from build123d import *

# Parameters (mm, degrees)
CHAMFER1_SIZE = 0.5


with BuildPart() as part:
    # Sketch1 → Revolve1 (revolve)
    with BuildSketch(Plane.XY, mode=Mode.PRIVATE) as revolve1_sk:
        with BuildLine():
            Line((5.5, 10.5), (2.236067977, 10.5))
            ThreePointArc((2.236067977, 10.5), (0, 9.5), (-2.236067977, 10.5))
            Line((-2.236067977, 10.5), (-5.5, 10.5))
            Line((-5.5, 10.5), (-5.5, 7.5))
            Line((-5.5, 7.5), (5.5, 7.5))
            Line((5.5, 7.5), (5.5, 10.5))
        make_face()
    revolve(revolve1_sk.sketch.rotate(Axis((-28.291139241, 0, 0), (1, 0, 0)), 90), axis=Axis((-28.291139241, 0, 0), (1, 0, 0)))

    # Chamfer1
    chamfer1_edges = [part.edges().sort_by_distance(p)[0] for p in [
        (-5.5, 0, -10.5),
        (5.5, 0, -10.5),
        (5.5, 0, -7.5),
        (-5.5, 0, -7.5),
    ]]
    chamfer(chamfer1_edges, length=CHAMFER1_SIZE)


solid = part.part
The listing builds one solid part. Answer for the finished solid, in the listing's coordinates (mm). Round coordinates to 2 decimals unless told otherwise and drop trailing zeros. Order: outer loops, then holes, each group sorted by start corner. A loop starts at its lowest first (then second) coordinate and runs counter-clockwise, first axis right, second up. Notation, with made-up numbers: M -10,45.25 L 24,45.25 A13 cw 24,62.25 Z; hole C -7.75,23.25 d7. An arc over 180 degrees is marked long. Answer in a Markdown table with one row per item. Add a question column.
1) The part is cut by section A-A on z = 0. Determine the outline of the cut face in (x, y).
2) Flat-ended cylindrical pins translate along their axes: pin 1 Ø10 at (y, z) = (-2.5, 5) entering from +X; pin 2 Ø2 at (x, z) = (-1.5, 5.5) entering from -Y; pin 3 Ø1 at (x, y) = (-3, 3.5) entering from +Z; pin 4 Ø1 at (x, z) = (-1.5, 1.5) entering from -Y. Find the tip coordinate at first contact, or state that the pin passes through.
3) The part is cut by section C-C on x = 1.25. Determine the outline of the cut face in (y, z), plus the area to 3 significant figures.
4) The part is cut by section B-B on x = -3.5. Determine the outline of the cut face in (y, z), plus the area to 3 significant figures.
5) Determine the mould class of faces 1 (the face through (-5.5, -8.2, 0)), 2 (the face through (3.6, -3.2, 10)), 3 (the face through (0.07, -6.324, 4.032)) for opening direction Z: pulls with the +Z half, pulls with the -Z half, needs draft (parallel to the pull), parting line crosses it, or undercut.
6) Consider line 1 along Z through (x, y) = (3, -2); line 2 along Z through (x, y) = (2.5, 6.75); line 3 along Y through (x, z) = (0.75, 0). Determine where each line is inside the solid, lowest interval first. Write a range as from..to.
Findings below:
| question | item | result |
|---|---|---|
| 1 | outline | M -5.5,-10 L -5,-10.5 L -2.24,-10.5 A3 cw 2.24,-10.5 L 5,-10.5 L 5.5,-10 L 5.5,-8 L 5,-7.5 L -5,-7.5 L -5.5,-8 Z; M -5.5,8 L -5,7.5 L 5,7.5 L 5.5,8 L 5.5,10 L 5,10.5 L 2.24,10.5 A3 cw -2.24,10.5 L -5,10.5 L -5.5,10 Z |
| 2 | pin 1 | stops at x = 5.5 |
| 2 | pin 2 | stops at y = -9.33 |
| 2 | pin 3 | stops at z = 10.06 |
| 2 | pin 4 | stops at y = -10.16 |
| 3 | outline | C 0,0 d19.55; hole C 0,0 d15 |
| 3 | area | 123 mm² |
| 4 | outline | C 0,0 d21; hole C 0,0 d15 |
| 4 | area | 170 mm² |
| 5 | face 1 | needs draft |
| 5 | face 2 | parting line crosses it |
| 5 | face 3 | undercut |
| 6 | line 1 | z = -10.31..-7.23, 7.23..10.31 |
| 6 | line 2 | z = -8.04..-3.27, 3.27..8.04 |
| 6 | line 3 | y = -9.6..-7.5, 7.5..9.6 |
